Can you work these out from the model? Positions are in its coordinate system, mm. Round coordinates to 2 decimals unless told otherwise and drop trailing zeros. Order: outer loops, then holes, each group sorted by start corner. A loop starts at its lowest first (then second) coordinate and runs counter-clockwise, first axis right, second up. Notation, with made-up numbers: M -27,25 L -12,25 A24 ccw -12,45 Z; hole C 61,-28 d10. An arc over 180 degrees is marked long. One line per question, with ' | ' between items.
```python
from build123d import *

# Parameters (mm, degrees)
SKETCH1_R           = 27.25
BOSS_EXTRUDE1_DEPTH = 5
SKETCH2_R           = 1.65
CUT_EXTRUDE1_DEPTH  = 10


with BuildPart() as part:
    # Sketch1 → Boss-Extrude1 (new body)
    with BuildSketch(Plane(origin=(0, 0, 0), x_dir=(1, 0, 0), z_dir=(0, 1, 0))):
        with Locations(Location((0, 0, 0), (0, 0, 270))):
            Circle(SKETCH1_R)
    extrude(amount=BOSS_EXTRUDE1_DEPTH)

    # Sketch2 → Cut-Extrude1 (cut)
    with BuildSketch(Plane(origin=(0, 5, 0), x_dir=(1, 0, 0), z_dir=(0, 1, 0))):
        with Locations(Location((0, 20, 0), (0, 0, 270))):
            Circle(SKETCH2_R)
        with Locations(Location((-16.383040886, 11.471528727, 0), (0, 0, 270))):
            Circle(SKETCH2_R)
        with Locations(Location((16.383040886, 11.471528727, 0), (0, 0, 270))):
            Circle(SKETCH2_R)
        with Locations(Location((16.383040886, -11.471528727, 0), (0, 0, 270))):
            Circle(SKETCH2_R)
        with Locations(Location((0, -20, 0), (0, 0, 270))):
            Circle(SKETCH2_R)
        with Locations(Location((-16.27093552, -11.629989565, 0), (0, 0, 270))):
            Circle(SKETCH2_R)
    extrude(amount=-CUT_EXTRUDE1_DEPTH, mode=Mode.SUBTRACT)


solid = part.part
```
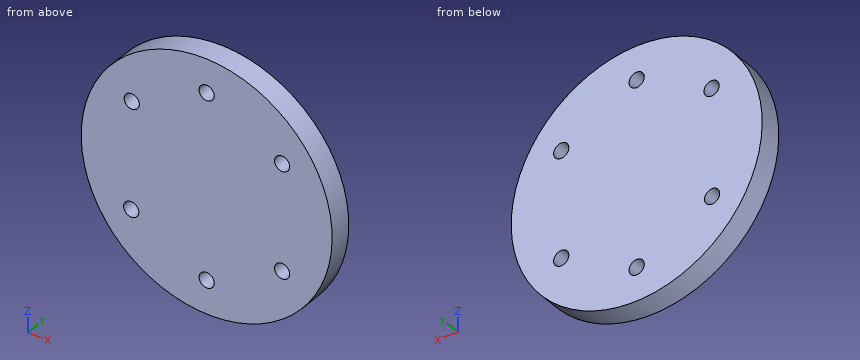
(1) If we section it at C-C on y = 1.85: Please give me the cut outline in (x, z).
Final values:
outline: C 0,0 d54.5; hole C -16.38,-11.47 d3.3; hole C -16.27,11.63 d3.3; hole C 0,-20 d3.3; hole C 0,20 d3.3; hole C 16.38,-11.47 d3.3; hole C 16.38,11.47 d3.3
(2) If we section it at D-D on z = 19: Please give me the cut outline in (x, y).
Final values:
outline: M -19.53,0 L -1.31,0 L -1.31,5 L -19.53,5 Z; M 1.31,0 L 19.53,0 L 19.53,5 L 1.31,5 Z
(3) If we section it at B-B on z = -12: Please give me the cut outline in (x, y).
Final values:
outline: M -24.47,0 L -17.95,0 L -17.95,5 L -24.47,5 Z; M -14.82,0 L 14.82,0 L 14.82,5 L -14.82,5 Z; M 17.95,0 L 24.47,0 L 24.47,5 L 17.95,5 Z
(4) If we section it at A-A on x = 0: Please give me the cut outline in (y, z), plus the area to 4 significant figures.
Final values:
outline: M 0,-27.25 L 5,-27.25 L 5,-21.65 L 0,-21.65 Z; M 0,-18.35 L 5,-18.35 L 5,18.35 L 0,18.35 Z; M 0,21.65 L 5,21.65 L 5,27.25 L 0,27.25 Z | area: 239.5 mm^2
(5) Will these pins go through, and if not, where does the flat tip stop? pin 1 Ø2 at (x, y) = (19, 4) entering from +Z; pin 2 Ø3 at (x, y) = (-13, 2.5) entering from -Z; pin 3 Ø2 at (x, y) = (-13.5, 2) entering from -Z.
Final values:
pin 1: z = 20.46 | pin 2: z = -24.7 | pin 3: z = -24.21
(6) Please list where these lines run through material, in increasing order: probe 1 along Z at (x, y) = (-15, 4.75); probe 2 along X at (y, z) = (1.45, 20); probe 3 along X at (y, z) = (3.05, 12). Write a range as [from, to].
Final values:
probe 1: [-22.75, -12.37], [-10.57, 10.58], [12.68, 22.75] | probe 2: [-18.51, -1.65], [1.65, 18.51] | probe 3: [-24.47, -17.88], [-14.66, 14.82], [17.95, 24.47]
